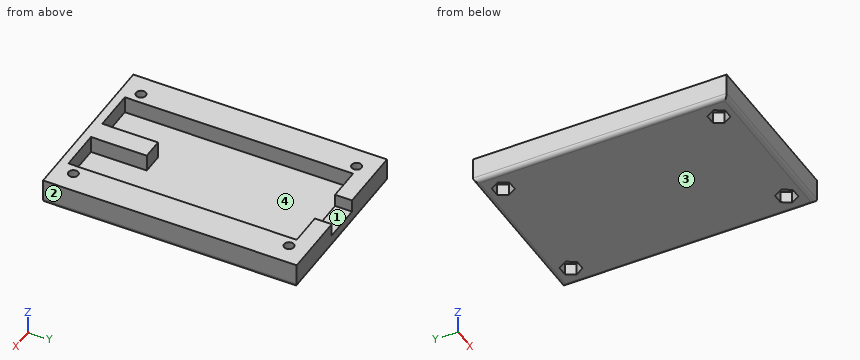
```python
from build123d import *

# Parameters (mm, degrees)
SKETCH1_W           = 60
SKETCH1_H           = 40
BOSS_EXTRUDE1_DEPTH = 6
SKETCH3_R           = 1.15
CUT_EXTRUDE2_DEPTH  = 73.360210061
SKETCH12_W          = 25
SKETCH12_H          = 40.8
CUT_EXTRUDE10_DEPTH = 4
CUT_EXTRUDE11_DEPTH = 2.8
FILLET1_R           = 1
SKETCH14_W          = 10
SKETCH14_H          = 13.2
CUT_EXTRUDE12_DEPTH = 4
SKETCH15_W          = 9
SKETCH15_H          = 4
CUT_EXTRUDE13_DEPTH = 3


with BuildPart() as part:
    # Sketch1 → Boss-Extrude1 (new body)
    with BuildSketch(Plane(origin=(0, 0, 0), x_dir=(0, 1, 0), z_dir=(0, 0, 1))):
        with Locations((30, -20)):
            Rectangle(SKETCH1_W, SKETCH1_H)
    extrude(amount=BOSS_EXTRUDE1_DEPTH)

    # Sketch3 → Cut-Extrude2 (cut, through all)
    with BuildSketch(Plane.XY.offset(6)):
        with Locations((5, 4.5)):
            Circle(SKETCH3_R)
        with Locations((35, 4.5)):
            Circle(SKETCH3_R)
        with Locations((5, 55.5)):
            Circle(SKETCH3_R)
        with Locations((35, 55.5)):
            Circle(SKETCH3_R)
    extrude(amount=-CUT_EXTRUDE2_DEPTH, mode=Mode.SUBTRACT)

    # Sketch12 → Cut-Extrude10 (cut)
    with BuildSketch(Plane.XY.offset(6)):
        with Locations((20, 35.6)):
            Rectangle(SKETCH12_W, SKETCH12_H)
    extrude(amount=-CUT_EXTRUDE10_DEPTH, mode=Mode.SUBTRACT)

    # Sketch13 → Cut-Extrude11 (cut)
    with BuildSketch(Plane(origin=(0, 0, 0), x_dir=(1, 0, 0), z_dir=(0, 0, -1))):
        Polygon((7.424871131, -55.5), (6.212435565, -53.4), (3.787564435, -53.4), (2.575128869, -55.5), (3.787564435, -57.6), (6.212435565, -57.6), align=None)
        Polygon((32.575128869, -55.5), (33.787564435, -57.6), (36.212435565, -57.6), (37.424871131, -55.5), (36.212435565, -53.4), (33.787564435, -53.4), align=None)
        Polygon((7.424871131, -4.5), (6.212435565, -2.4), (3.787564435, -2.4), (2.575128869, -4.5), (3.787564435, -6.6), (6.212435565, -6.6), align=None)
        Polygon((32.575128869, -4.5), (33.787564435, -6.6), (36.212435565, -6.6), (37.424871131, -4.5), (36.212435565, -2.4), (33.787564435, -2.4), align=None)
    extrude(amount=-CUT_EXTRUDE11_DEPTH, mode=Mode.SUBTRACT)

    # Fillet1
    fillet1_edges = [part.edges().sort_by_distance(p)[0] for p in [
        (0, 30, 0),
        (20, 60, 0),
        (40, 30, 0),
        (20, 0, 0),
    ]]
    fillet(fillet1_edges, radius=FILLET1_R)

    # Sketch14 → Cut-Extrude12 (cut)
    with BuildSketch(Plane.XY.offset(6)):
        with Locations((12.5, 8.6)):
            Rectangle(SKETCH14_W, SKETCH14_H)
        with Locations((27.5, 8.6)):
            Rectangle(SKETCH14_W, SKETCH14_H)
    extrude(amount=-CUT_EXTRUDE12_DEPTH, mode=Mode.SUBTRACT)

    # Sketch15 → Cut-Extrude13 (cut)
    with BuildSketch(Plane.XY.offset(6)):
        with Locations((20, 58)):
            Rectangle(SKETCH15_W, SKETCH15_H)
    extrude(amount=-CUT_EXTRUDE13_DEPTH, mode=Mode.SUBTRACT)


solid = part.part
```
Here's how the part is built. I have some questions about the finished solid (model axes, mm). Face numbers are marked on the shaded views. A direction names the side the tool comes from. Round coordinates to 2 decimals unless told otherwise and drop trailing zeros. Loops run counter-clockwise (first coordinate to the right, second up) from the corner with the lowest first, then second, coordinate; pieces in that order, holes last. Notation, with made-up numbers: (-26, 6) -> (19, 6) arc R26 ccw to (19, 38) -> close; hole circle Ø5 at (10, 52). An arc over 180 degrees is marked (long way). Answer as CSV lines item,"result".
1. Thinking about a two-plate mould opening in Y: for the marked faces 3 and 4, which applies, released by +Y, released by -Y, zero draft, split by the parting line, or undercut?
Final values:
face 3,"zero draft"
face 4,"undercut"
2. Which directions (+Z, -Z, +X, -X, +Y, -Y) give clear straight access to the entire face, cutting with the end or side of a thin tool? Please do the marked faces 1 and 2.
Final values:
face 1,"+Z, +Y"
face 2,"+Z, -Z, +X, +Y, -Y"
3. If we section it at C-C on y = 44: Please give me the cut outline in (x, z), plus the area to 3 significant figures.
Final values:
outline,"(0, 1) arc R1 ccw to (1, 0) -> (39, 0) arc R1 ccw to (40, 1) -> (40, 6) -> (32.5, 6) -> (32.5, 2) -> (7.5, 2) -> (7.5, 6) -> (0, 6) -> close"
area,"140 mm^2"
4. If I drill on L1, parallel to X at y = 8, z = 4.9; L2, parallel to Y at x = 35, z = 4.6; L3, parallel to X at y = 54.5, z = 3.75, over which ranges is the centre line in solid material (lowest first)?
Final values:
L1,"x = 0 to 7.5, 17.5 to 22.5, 32.5 to 40"
L2,"y = 0 to 3.35, 5.65 to 54.35, 56.65 to 60"
L3,"x = 0 to 4.43, 5.57 to 7.5, 32.5 to 34.43, 35.57 to 40"
5. If we section it at B-B on z = 4.15: Please give me the cut outline in (x, y).
Final values:
outline,"(0, 0) -> (40, 0) -> (40, 60) -> (24.5, 60) -> (24.5, 56) -> (32.5, 56) -> (32.5, 2) -> (22.5, 2) -> (22.5, 15.2) -> (17.5, 15.2) -> (17.5, 2) -> (7.5, 2) -> (7.5, 56) -> (15.5, 56) -> (15.5, 60) -> (0, 60) -> close; hole circle Ø2.3 at (5, 4.5); hole circle Ø2.3 at (5, 55.5); hole circle Ø2.3 at (35, 4.5); hole circle Ø2.3 at (35, 55.5)"
6. If we section it at D-D on x = 30.5: Please give me the cut outline in (y, z), plus the area to 3 significant figures.
Final values:
outline,"(0, 1) arc R1 ccw to (1, 0) -> (59, 0) arc R1 ccw to (60, 1) -> (60, 6) -> (56, 6) -> (56, 2) -> (2, 2) -> (2, 6) -> (0, 6) -> close"
area,"144 mm^2"
7. If we section it at A-A on x = 5: Please give me the cut outline in (y, z), plus the area to 3 significant figures.
Final values:
outline,"(0, 1) arc R1 ccw to (1, 0) -> (2.4, 0) -> (2.4, 2.8) -> (3.35, 2.8) -> (3.35, 6) -> (0, 6) -> close; (5.65, 2.8) -> (6.6, 2.8) -> (6.6, 0) -> (53.4, 0) -> (53.4, 2.8) -> (54.35, 2.8) -> (54.35, 6) -> (5.65, 6) -> close; (56.65, 2.8) -> (57.6, 2.8) -> (57.6, 0) -> (59, 0) arc R1 ccw to (60, 1) -> (60, 6) -> (56.65, 6) -> close"
area,"321 mm^2"
8. For pin 1 (1.2 mm diameter, centred on x = 19, y = 57.5, fed in from +Z); pin 2 (2.5 mm diameter, centred on x = 5, z = 1.5, fed in from -Y); pin 3 (2 mm diameter, centred on x = 4.5, y = 4, fed in from -Z); pin 4 (1.2 mm diameter, centred on x = 20.5, z = 4, fed in from +Y), each with a flat end and sliding along its axis, tell me the tip position at first contact or that it passes through.
Final values:
pin 1,"stops at z = 3"
pin 2,"stops at y = 0"
pin 3,"stops at z = 2.8"
pin 4,"stops at y = 15.2"
